Source: CAD feature listing. Evaluate the final solid. Frame: model axes, mm. Face numbers are marked on the shaded views. A direction names the side the tool comes from. Give positions to 0.01 mm unless a question says otherwise; leave off trailing zeros. Order: outer loops, then holes, each group sorted by start corner. A loop starts at its lowest first (then second) coordinate and runs counter-clockwise, first axis right, second up.
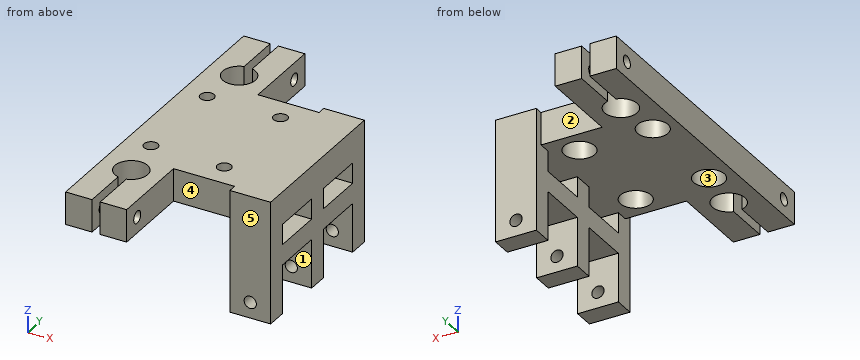
from build123d import *

# Parameters (mm, degrees)
SKETCH_1_W          = 30
SKETCH_1_H          = 36
SKETCH_1_R          = 1.7
EXTRUDE_1_DEPTH     = 8
SKETCH_2_R          = 3.75
CUT_EXTRUDE_1_DEPTH = 4.5
SKETCH_3_W          = 15
SKETCH_3_H          = 20
SKETCH_3_R          = 4
EXTRUDE_4_DEPTH     = 8
SKETCH_8_W          = 10
SKETCH_8_H          = 40
EXTRUDE_5_DEPTH     = 30
SKETCH_10_W         = 12
SKETCH_10_H         = 12.5
SKETCH_10_W_2       = 5
CUT_EXTRUDE_4_DEPTH = 30
SKETCH_11_R         = 1.5
CUT_EXTRUDE_5_DEPTH = 47
SKETCH_12_W         = 2
SKETCH_12_H         = 25.842259392
SKETCH_12_H_2       = 30.756424204
CUT_EXTRUDE_6_DEPTH = 10
SKETCH_13_R         = 1.5
CUT_EXTRUDE_7_DEPTH = 40


with BuildPart() as part:
    # 草图1 → 凸台-拉伸1 (new body)
    with BuildSketch(Plane.XY):
        with Locations((-3.375, -1.625)):
            Rectangle(SKETCH_1_W, SKETCH_1_H)
        with Locations((-12.375, 10.375)):
            Circle(SKETCH_1_R, mode=Mode.SUBTRACT)
        with Locations((-12.375, -13.625)):
            Circle(SKETCH_1_R, mode=Mode.SUBTRACT)
        with Locations(Location((5.625, -13.625, 0), (0, 0, 180))):
            Circle(SKETCH_1_R, mode=Mode.SUBTRACT)
        with Locations(Location((5.625, 10.375, 0), (0, 0, 180))):
            Circle(SKETCH_1_R, mode=Mode.SUBTRACT)
    extrude(amount=EXTRUDE_1_DEPTH)

    # 草图2 → 切除-拉伸1 (cut)
    with BuildSketch(Plane(origin=(0, 0, 0), x_dir=(-1, 0, 0), z_dir=(0, 0, -1))):
        with Locations((12.375, 10.375)):
            Circle(SKETCH_2_R)
        with Locations(Location((-5.625, 10.375, 0), (0, 0, 180))):
            Circle(SKETCH_2_R)
        with Locations(Location((12.375, -13.625, 0), (0, 0, 180))):
            Circle(SKETCH_2_R)
        with Locations((-5.625, -13.625)):
            Circle(SKETCH_2_R)
    extrude(amount=-CUT_EXTRUDE_1_DEPTH, mode=Mode.SUBTRACT)

    # 草图3 → 凸台-拉伸4 (add)
    # profile 1 of 2: a face of its own
    with BuildSketch(Plane.XY.offset(8)):
        with Locations((-10.875, 26.375)):
            Rectangle(SKETCH_3_W, SKETCH_3_H)
        with Locations((-10.875, 21.375)):
            Circle(SKETCH_3_R, mode=Mode.SUBTRACT)
    # profile 2 of 2: a face of its own
    with BuildSketch(Plane.XY.offset(8)):
        with Locations((-10.875, -29.625)):
            Rectangle(SKETCH_3_W, SKETCH_3_H)
        with Locations((-10.875, -24.625)):
            Circle(SKETCH_3_R, mode=Mode.SUBTRACT)
    extrude(amount=-EXTRUDE_4_DEPTH)

    # 草图8 → 凸台-拉伸5 (add)
    with BuildSketch(Plane.XY.offset(8)):
        with Locations((16.625, -1.625)):
            Rectangle(SKETCH_8_W, SKETCH_8_H)
    extrude(amount=-EXTRUDE_5_DEPTH)

    # 草图10 → 切除-拉伸4 (cut)
    with BuildSketch(Plane.ZY.offset(-11.625)):
        with Locations((-16, 7.125)):
            Rectangle(SKETCH_10_W, SKETCH_10_H)
        with Locations((-2.5, 7.125)):
            Rectangle(SKETCH_10_W_2, SKETCH_10_H)
        with Locations((-2.5, -10.375)):
            Rectangle(SKETCH_10_W_2, SKETCH_10_H)
        with Locations((-16, -10.375)):
            Rectangle(SKETCH_10_W, SKETCH_10_H)
    extrude(amount=-CUT_EXTRUDE_4_DEPTH, mode=Mode.SUBTRACT)

    # 草图11 → 切除-拉伸5 (cut)
    with BuildSketch(Plane(origin=(0, 18.375, 0), x_dir=(1, 0, 0), z_dir=(0, 1, 0))):
        with Locations(Location((16.621809271, 18.123313308, 0), (0, 0, 180))):
            Circle(SKETCH_11_R)
    extrude(amount=-CUT_EXTRUDE_5_DEPTH, mode=Mode.SUBTRACT)

    # 草图12 → 切除-拉伸6 (cut)
    with BuildSketch(Plane(origin=(0, 0, 0), x_dir=(-1, 0, 0), z_dir=(0, 0, -1))):
        with Locations((10.875, 36.375)):
            Rectangle(SKETCH_12_W, SKETCH_12_H)
        with Locations((10.875, -39.625)):
            Rectangle(SKETCH_12_W, SKETCH_12_H_2)
    extrude(amount=-CUT_EXTRUDE_6_DEPTH, mode=Mode.SUBTRACT)

    # 草图13 → 切除-拉伸7 (cut)
    with BuildSketch(Plane.ZY.offset(18.375)):
        with Locations((3.892451488, 31.868119268)):
            Circle(SKETCH_13_R)
        with Locations(Location((3.892451488, -35.118119268, 0), (0, 0, 270))):
            Circle(SKETCH_13_R)
    extrude(amount=-CUT_EXTRUDE_7_DEPTH, mode=Mode.SUBTRACT)


solid = part.part
1) First-contact query: pin 1 Ø6 at (y, z) = (5.5, -7.5) entering from -X (3 decimals); pin 2 Ø5 at (x, z) = (10.5, -16.5) entering from -Y (3 decimals); pin 3 Ø4 at (x, z) = (16.62, -18.12) entering from +Y (3 decimals). Flat tips, straight axial feed; report the tip coordinate or a pass-through.
Checks:
pin 1: stops at x = 11.625
pin 2: stops at y = -21.625
pin 3: stops at y = 18.375
2) Section query A-A on y = 29. Output: boundary loops of the cut face in (x, z) (3 decimals).
Checks:
outline: (-18.375, 0) - (-11.875, 0) - (-11.875, 8) - (-18.375, 8) - close; (-9.875, 0) - (-3.375, 0) - (-3.375, 8) - (-9.875, 8) - close
3) Section query D-D on y = -26.5. Output: boundary loops of the cut face in (x, z) (3 decimals), and give its area (3 significant figures).
Checks:
outline: (-18.375, 0) - (-14.408, 0) - (-14.408, 8) - (-18.375, 8) - close; (-7.342, 0) - (-3.375, 0) - (-3.375, 8) - (-7.342, 8) - close
area: 63.5 mm2
4) Section query C-C on x = 6.5. Output: boundary loops of the cut face in (y, z) (3 decimals).
Checks:
outline: (-19.625, 0) - (-17.271, 0) - (-17.271, 4.5) - (-15.083, 4.5) - (-15.083, 8) - (-19.625, 8) - close; (-12.167, 4.5) - (-9.979, 4.5) - (-9.979, 0) - (6.729, 0) - (6.729, 4.5) - (8.917, 4.5) - (8.917, 8) - (-12.167, 8) - close; (11.833, 4.5) - (14.021, 4.5) - (14.021, 0) - (16.375, 0) - (16.375, 8) - (11.833, 8) - close
5) Section query B-B on z = -15.25. Output: boundary loops of the cut face in (x, y) (3 decimals), and give its area (3 significant figures).
Checks:
outline: (11.625, -21.625) - (21.625, -21.625) - (21.625, -16.625) - (11.625, -16.625) - close; (11.625, -4.125) - (21.625, -4.125) - (21.625, 0.875) - (11.625, 0.875) - close; (11.625, 13.375) - (21.625, 13.375) - (21.625, 18.375) - (11.625, 18.375) - close
area: 150 mm2
6) Ray query, L1, parallel to Y at x = 15.5, z = -20 (3 decimals); L2, parallel to Z at x = -11, y = -8; L3, parallel to X at y = -31, z = 1.25 (3 decimals). Return the intervals inside material, ascending.
Checks:
L1: y = -21.625 to -16.625, -4.125 to 0.875, 13.375 to 18.375
L2: z = 0 to 8
L3: x = -18.375 to -11.875, -9.875 to -3.375
7) Reachability of the marked faces 1, 2, 3, 4 and 5 from +Z, -Z, +X, -X, +Y, -Y: full face, straight path, thin tool, end or side. Return the list, or none.
Checks:
face 1: -Z, +X, -X
face 2: +Z, -Z, +Y
face 3: -Z
face 4: +Z, -Z, -Y
face 5: +Z, -Z, +X, -Y
